Autodesk Inventor part; units mm, degrees
ref_plane "Work Plane1" through (2733.5993, 510.3823, 544.9206) normal (0.1045285, 0, 0.9945219) x (0.0000001, 1, 0)
ref_plane "Work Plane3" through (2730.0713, 509.1816, 518.0623) normal (0.3805886, 0.9238789, -0.0400015) x (-0.9188178, 0.382685, 0.0965716)
ref_plane "YZ Plane" through (0, 0, 0) normal (1, 0, 0) x (0, 1, 0)
ref_plane "Work Plane1" through (2733.5993, 510.3823, 544.9206) normal (0.1045285, 0, 0.9945219) x (0.0000001, 1, 0)
sketch "Sketch1" plane through (2733.5993, 510.3823, 544.9206) normal (0.1045285, 0, 0.9945219) x (0.0000001, 1, 0)
  circle A0 centre (0, 3.6) radius 3.85
  line L0 (-510.3825, -1.79) -> (-510.3825, 8.99)
  line L1 (-5.3902, 2661.6646) -> (5.3898, 2661.6646)
  line L2 (-510.3824, 8.99) -> (-510.3824, -1.79)
  dimension "d0" = 7.7
  dimension "d1" = 510.3825
  dimension "d2" = 2658.0646
extrude "Extrusion1" add sketch "Sketch1" against normal blind 5
sketch "Sketch2" plane through (2729.4964, 510.3823, 540.3243) normal (-0.1045285, 0, -0.9945219) x (-0.9945219, 0, 0.1045285)
  circle A0 centre (0, 0) radius 3.85
  circle A1 centre (0, 0) radius 4.9459
  dimension "d5" = 9.8917
extrude "Extrusion2" add sketch "Sketch2" along normal blind 22.08 contours A0 | A1
sketch "Sketch3" plane through (2727.1884, 510.3823, 518.3653) normal (-0.1045285, 0, -0.9945219) x (-0.9945219, 0, 0.1045285)
  circle A0 centre (0, 0) radius 4.9459
  line L0 (0, -8.1991) -> (-5.7976, -5.7977)
  line L1 (-5.7976, -5.7977) -> (-8.1991, 0)
  line L2 (-8.1991, 0) -> (-5.7977, 5.7976)
  line L3 (-5.7977, 5.7976) -> (0, 8.1991)
  line L4 (0, 8.1991) -> (5.7976, 5.7977)
  line L5 (5.7976, 5.7977) -> (8.1991, 0)
  line L6 (8.1991, 0) -> (5.7977, -5.7976)
  line L7 (5.7977, -5.7976) -> (0, -8.1991)
  line L8 (-12.0322, -510.3825) -> (14.7999, -510.3825)
  line L9 (2658.0646, -11.4788) -> (2658.0646, 11.4788)
  line L10 (14.7999, -510.3823) -> (-12.0323, -510.3823)
  dimension "d8" = 5.7976
  dimension "d9" = 2.4015
extrude "Extrusion3" add sketch "Sketch3" along normal blind 1.8 contours A0 | L0 L1 L2 L3 L4 L5 L6 L7
sketch "Sketch4" plane through (2727.0002, 510.3823, 516.5751) normal (-0.1045285, 0, -0.9945219) x (-0.9945219, 0, 0.1045285)
  circle A0 centre (0, 0) radius 6.3211
  line L0 (-12.2942, -510.3825) -> (15.0619, -510.3825)
  line L1 (2658.0646, -11.4788) -> (2658.0646, 11.4788)
  line L2 (15.0619, -510.3823) -> (-12.2942, -510.3823)
  dimension "d12" = 12.6421
  dimension "d14" = 510.3823
  dimension "d15" = 2658.0646
extrude "Extrusion4" add sketch "Sketch4" along normal blind 0.7
sketch "Sketch5" plane through (2726.927, 510.3823, 515.879) normal (-0.1045285, 0, -0.9945219) x (-0.9945219, 0, 0.1045285)
  circle A0 centre (0, 0) radius 6.3211
  circle A1 centre (0, 0) radius 9.5
  dimension "d18" = 19
extrude "Extrusion5" add sketch "Sketch5" along normal blind 3 contours A0 | A1
fillet "Fillet1" radius 3 1 edges at (2736.0614, 510.3823, 511.9024)
fillet "Fillet1" radius 1 1 edges at (2733.2866, 510.3823, 515.9144)
fillet "Fillet1" radius 0.5 1 edges at (2732.1071, 510.3823, 517.8483)
fillet "Fillet1" radius 0.25 1 edges at (2730.019, 506.5323, 545.2969)
sketch "Sketch6" plane through (2726.6135, 510.3823, 512.8954) normal (-0.1045285, 0, -0.9945219) x (-0.9945219, 0, 0.1045285)
  circle A0 centre (0, 0) radius 6.5
  circle A1 centre (0, 0) radius 5
  dimension "d25" = 10
extrude "Extrusion6" cut sketch "Sketch6" against normal blind 2 contours A1
fillet "Fillet2" radius 0.5 1 edges at (2731.7953, 510.3823, 514.3638)
chamfer "Chamfer2" distance 0.3766 angle 45 1 edges at (2727.0943, 502.1832, 517.4702)
chamfer "Chamfer3" distance 0.3766 angle 45 1 edges at (2732.8602, 504.5847, 516.8642)
chamfer "Chamfer4" distance 0.3766 angle 45 1 edges at (2735.2485, 510.3823, 516.6132)
chamfer "Chamfer5" distance 0.3766 angle 45 1 edges at (2732.8602, 516.18, 516.8642)
chamfer "Chamfer6" distance 0.3766 angle 45 1 edges at (2727.0943, 518.5815, 517.4702)
chamfer "Chamfer7" distance 0.3766 angle 45 1 edges at (2721.3284, 516.18, 518.0762)
chamfer "Chamfer8" distance 0.3766 angle 45 1 edges at (2718.9401, 510.3824, 518.3272)
chamfer "Chamfer9" distance 0.3766 angle 45 1 edges at (2721.3284, 504.5847, 518.0762)
ref_plane "Work Plane3" through (2730.0713, 509.1816, 518.0623) normal (0.3805886, 0.9238789, -0.0400015) x (-0.9188178, 0.382685, 0.0965716)
ref_plane "Work Plane2" through (2732.9543, 516.18, 517.7593) normal (0.3805886, 0.9238789, -0.0400015) x (-0.9188178, 0.382685, 0.0965716)
chamfer "Chamfer10" distance 1.095 distance2 1.298 1 edges at (2734.4151, 510.3823, 539.8073) measured on face at (2728.4119, 514.8065, 540.4383)
thread "Thread1"
properties part number "314-10" material "Steel, Mild"
Geometry: final body of the model. Coordinates: model frame, mm. A direction names the side the tool comes from. Give positions to 0.01 mm unless a question says otherwise; leave off trailing zeros. Return JSON: item names as keys, results as strings. Group by question number.
1) Mould query, pull axis Y, two halves, no side actions, for faces 6 (the cylindrical face through (2728.598, 514.055, 542.84)), 7 (the cylindrical face through (2730.637, 507.34, 513.217)), 8 (the flat face through (2734.04, 507.45, 516.75)). Classes: released by +Y, released by -Y, zero draft, split by the parting line, or undercut.
2) First-contact query: P1, Ø1, axis at x = 2724, z = 535, coming from the -Y side; P2, Ø4, axis at y = 507, z = 539, coming from the -X side; P3, Ø2, axis at x = 2730.5, z = 522.5, coming from the -Y side; P4, Ø10, axis at x = 2732.5, y = 511.5, coming from the -Z side. Flat tips, straight axial feed; report the tip coordinate or a pass-through.
3) Line query: line 1 (Z direction, x = 2728.75, y = 503); line 2 (Y direction, x = 2724.5, z = 515); line 3 (Z direction, x = 2729.25, y = 503). Output: solid intervals per line, ascending.
4) Set-up query: faces 1 (the flat face through (2730.014, 517.366, 517.176)), 2 (the flat face through (2730, 510.3, 545.3)), 3 (the flat face through (2720.761, 508.404, 516.527)), 4 (the flat face through (2729.94, 503.37, 517.18)), 5 (the flat face through (2726.89, 510.45, 514.88)). Return all of +Z, -Z, +X, -X, +Y, -Y with unobstructed straight access to the full face (end or side cutting, diameter ignored); none if empty.
Filled in:
{
 "1": {"face 6": "split by the parting line", "face 7": "undercut", "face 8": "released by -Y"},
 "2": {"P1": "stops at y = 508.14", "P2": "stops at x = 2724.55", "P3": "stops at y = 505.8", "P4": "stops at z = 512.2"},
 "3": {"line 1": "z = 512.91 to 515.69, 516.39 to 518.2", "line 2": "y = 501.4 to 506.14, 514.62 to 519.37", "line 3": "z = 512.93 to 515.63"},
 "4": {"face 1": "+X, +Y", "face 2": "+Z, +X, +Y, -Y", "face 3": "none", "face 4": "+X, -Y", "face 5": "-Z"}
}
